The listing builds one solid part. Answer for the finished solid, in the listing's coordinates (mm). Give positions to 0.01 mm unless a question says otherwise; leave off trailing zeros. Write each loop counter-clockwise with the first axis right and the second up, starting at its lowest first coordinate (ties: lowest second). Pieces come first, ordered by that corner, then holes. Notation, with made-up numbers: (83, 86.25) - (97, 86.25) arc R19 cw to (97, 112.25) - close; hole circle Ø6 at (50, 12.5). An arc over 180 degrees is marked (long way). Write each question's results on one line, items separated by ' | '. Start each with the question number.
Q1. A flat-ended cylindrical pin translates along its axis: pin 1 Ø0.5 at (x, z) = (25, 1) entering from -Y. Find the tip coordinate at first contact, or state that the pin passes through.
Q2. Find the intervals of material crossed by probe 1 along Y at (x, z) = (13, 0.4); probe 2 along X at (y, z) = (-3, 0.8), in increasing order.
Q3. Section C-C (x = 20) is taken. Determine the outline of the cut face in (y, z).
Q4. Section B-B (y = -2.25) is taken. Determine the outline of the cut face in (x, z).
Q5. Section A-A (z = 0.7) is taken. Determine the outline of the cut face in (x, y).
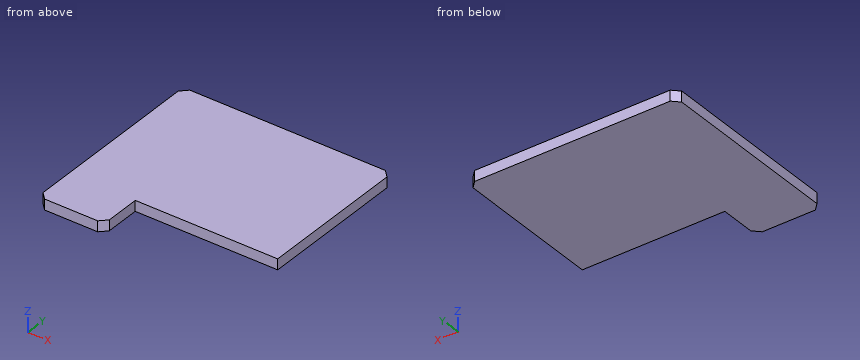
```python
from build123d import *

# Parameters (mm, degrees)
BOX002_W        = 31.5
BOX002_H        = 23.3
BOX002_DEPTH    = 1.6
CHAMFER001_SIZE = 1
BOX003_W        = 10
BOX003_H        = 6.3
BOX003_DEPTH    = 1.6
CHAMFER_SIZE    = 1


with BuildPart() as chamfer001:
    # Box002 → Box002 (new body)
    with BuildSketch(Plane.XY):
        with Locations((15.75, 11.65)):
            Rectangle(BOX002_W, BOX002_H)
    extrude(amount=BOX002_DEPTH)

    # Chamfer001
    chamfer001_edges = [chamfer001.edges().sort_by_distance(p)[0] for p in [
        (0, 23.3, 0.8),
        (31.5, 23.3, 0.8),
    ]]
    chamfer(chamfer001_edges, length=CHAMFER001_SIZE)


with BuildPart() as obj1:
    # Box003 → Box003 (new body)
    with BuildSketch(Plane(origin=(0, -6.3, 0), x_dir=(1, 0, 0), z_dir=(0, 0, 1))):
        with Locations((5, 3.15)):
            Rectangle(BOX003_W, BOX003_H)
    extrude(amount=BOX003_DEPTH)

    # Chamfer
    chamfer_edges = [obj1.edges().sort_by_distance(p)[0] for p in [
        (0, -6.3, 0.8),
        (10, -6.3, 0.8),
    ]]
    chamfer(chamfer_edges, length=CHAMFER_SIZE)

    # Fusion: union Chamfer001
    add(chamfer001.part)


solid = obj1.part
```
Answers below:
1) pin 1: stops at y = 0
2) probe 1: y = 0 to 23.3 | probe 2: x = 0 to 10
3) outline: (0, 0) - (23.3, 0) - (23.3, 1.6) - (0, 1.6) - close
4) outline: (0, 0) - (10, 0) - (10, 1.6) - (0, 1.6) - close
5) outline: (0, -5.3) - (1, -6.3) - (9, -6.3) - (10, -5.3) - (10, 0) - (31.5, 0) - (31.5, 22.3) - (30.5, 23.3) - (1, 23.3) - (0, 22.3) - close
